CAD build for the part. Positions are in the model's coordinates, mm. A direction names the side the tool comes from. Round coordinates to 2 decimals unless told otherwise and drop trailing zeros. Loops run counter-clockwise (first coordinate to the right, second up) from the corner with the lowest first, then second, coordinate; pieces in that order, holes last.
```python
from build123d import *

# Parameters (mm, degrees)
SKETCH_1_W          = 40
SKETCH_1_H          = 2.5
EXTRUDE_1_DEPTH     = 18.5
SKETCH_2_R          = 1.5
CUT_EXTRUDE_1_DEPTH = 33.958808433
SKETCH_3_R          = 1.5
CUT_EXTRUDE_2_DEPTH = 40
SKETCH_4_W          = 40
SKETCH_4_H          = 5.719865779
CUT_EXTRUDE_3_DEPTH = 40
SKETCH_5_W          = 40
SKETCH_5_H          = 12.780134221
EXTRUDE_2_DEPTH     = 1
SKETCH_6_R          = 1.5
CUT_EXTRUDE_4_DEPTH = 31.221927206
SKETCH_8_W          = 40
SKETCH_8_H          = 3.5
EXTRUDE_3_DEPTH     = 5
SKETCH_9_R          = 3.8
CUT_EXTRUDE_5_DEPTH = 1
SKETCH_10_W         = 12
SKETCH_10_H         = 17.780134221
CUT_EXTRUDE_6_DEPTH = 1.5
CHAMFER_3_SIZE      = 0.7
CUT_EXTRUDE_7_DEPTH = 31.221927206
SKETCH_12_W         = 40
SKETCH_12_H         = 1.953894505
EXTRUDE_5_DEPTH     = 2
SKETCH_13_W         = 40
SKETCH_13_H         = 3.5
EXTRUDE_6_DEPTH     = 5
SKETCH_14_W         = 12
SKETCH_14_H         = 4.371099825
EXTRUDE_7_DEPTH     = 2
SKETCH_15_W         = 12
SKETCH_15_H         = 1.544999831
EXTRUDE_8_DEPTH     = 2


with BuildPart() as part:
    # Эскиз1 → Бобышка-Вытянуть1 (new body)
    with BuildSketch(Plane(origin=(0, 0, 0), x_dir=(1, 0, 0), z_dir=(0, 1, 0))):
        with Locations((7.162162162, 1.25)):
            Rectangle(SKETCH_1_W, SKETCH_1_H)
    extrude(amount=EXTRUDE_1_DEPTH)

    # Эскиз2 → Вырез-Вытянуть1 (cut, through all)
    with BuildSketch(Plane.XY):
        with Locations((-6.837837838, 3)):
            Circle(SKETCH_2_R)
        with Locations((21.162162162, 3)):
            Circle(SKETCH_2_R)
    extrude(amount=-CUT_EXTRUDE_1_DEPTH, mode=Mode.SUBTRACT)

    # Эскиз3 → Вырез-Вытянуть2 (cut)
    with BuildSketch(Plane.XY):
        with Locations((-2.337837838, 9.3)):
            Circle(SKETCH_3_R)
        with Locations((17.662162162, 9.3)):
            Circle(SKETCH_3_R)
    extrude(amount=-CUT_EXTRUDE_2_DEPTH, mode=Mode.SUBTRACT)

    # Эскиз4 → Вырез-Вытянуть3 (cut)
    with BuildSketch(Plane.XY):
        with Locations((7.162162162, 15.640067111)):
            Rectangle(SKETCH_4_W, SKETCH_4_H)
    extrude(amount=-CUT_EXTRUDE_3_DEPTH, mode=Mode.SUBTRACT)

    # Эскиз5 → Бобышка-Вытянуть2 (add)
    with BuildSketch(Plane.XY):
        with Locations((7.162162162, 6.390067111)):
            Rectangle(SKETCH_5_W, SKETCH_5_H)
    extrude(amount=EXTRUDE_2_DEPTH)

    # Эскиз6 → Вырез-Вытянуть4 (cut, through all)
    with BuildSketch(Plane(origin=(0, 0, -2.5), x_dir=(-1, 0, 0), z_dir=(0, 0, -1))):
        with Locations(Location((-17.662162162, 9.3, 0), (0, 0, 180))):
            Circle(SKETCH_6_R)
        with Locations(Location((2.337837838, 9.3, 0), (0, 0, 180))):
            Circle(SKETCH_6_R)
        with Locations(Location((6.837837838, 3, 0), (0, 0, 180))):
            Circle(SKETCH_6_R)
        with Locations(Location((-21.162162162, 3, 0), (0, 0, 180))):
            Circle(SKETCH_6_R)
    extrude(amount=-CUT_EXTRUDE_4_DEPTH, mode=Mode.SUBTRACT)

    # Эскиз8 → Бобышка-Вытянуть3 (add)
    with BuildSketch(Plane.XZ):
        with Locations((7.162162162, -0.75)):
            Rectangle(SKETCH_8_W, SKETCH_8_H)
    extrude(amount=EXTRUDE_3_DEPTH)

    # Эскиз9 → Вырез-Вытянуть5 (cut)
    with BuildSketch(Plane.XY.offset(1)):
        with Locations((-6.837837838, 3)):
            Circle(SKETCH_9_R)
        with Locations((21.162162162, 3)):
            Circle(SKETCH_9_R)
    extrude(amount=-CUT_EXTRUDE_5_DEPTH, mode=Mode.SUBTRACT)

    # Эскиз10 → Вырез-Вытянуть6 (cut)
    with BuildSketch(Plane(origin=(0, 0, -2.5), x_dir=(-1, 0, 0), z_dir=(0, 0, -1))):
        with Locations((-7.662162162, 3.890067111)):
            Rectangle(SKETCH_10_W, SKETCH_10_H)
    extrude(amount=-CUT_EXTRUDE_6_DEPTH, mode=Mode.SUBTRACT)

    # Фаска3
    chamfer_3_edges = [part.edges().sort_by_distance(p)[0] for p in [
        (-10.637837838, 3, 0),
        (17.362162162, 3, 0),
    ]]
    chamfer(chamfer_3_edges, length=CHAMFER_3_SIZE)

    # Эскиз11 → Вырез-Вытянуть7 (cut, through all)
    with BuildSketch(Plane.XY.offset(1)):
        Polygon((-12.837837838, 12.780134221), (-12.837837838, 7.280134221), (-7.337837838, 12.780134221), align=None)
        Polygon((27.162162162, 12.780134221), (21.662162162, 12.780134221), (27.162162162, 7.280134221), align=None)
    extrude(amount=-CUT_EXTRUDE_7_DEPTH, mode=Mode.SUBTRACT)

    # Эскиз12 → Бобышка-Вытянуть5 (add)
    with BuildSketch(Plane.XY.offset(1)):
        with Locations((7.162162162, 6.303186969)):
            Rectangle(SKETCH_12_W, SKETCH_12_H)
    extrude(amount=-EXTRUDE_5_DEPTH)

    # Эскиз13 → Бобышка-Вытянуть6 (add)
    with BuildSketch(Plane.XZ.offset(5)):
        with Locations((7.162162162, -0.75)):
            Rectangle(SKETCH_13_W, SKETCH_13_H)
    extrude(amount=EXTRUDE_6_DEPTH)

    # Эскиз14 → Бобышка-Вытянуть7 (add)
    with BuildSketch(Plane(origin=(0, 0, -2.5), x_dir=(-1, 0, 0), z_dir=(0, 0, -1))):
        with Locations((-7.662162162, -2.814450088)):
            Rectangle(SKETCH_14_W, SKETCH_14_H)
    extrude(amount=-EXTRUDE_7_DEPTH)

    # Эскиз15 → Бобышка-Вытянуть8 (add)
    with BuildSketch(Plane(origin=(0, 0, -2.5), x_dir=(-1, 0, 0), z_dir=(0, 0, -1))):
        with Locations((-7.662162162, 12.007634306)):
            Rectangle(SKETCH_15_W, SKETCH_15_H)
    extrude(amount=-EXTRUDE_8_DEPTH)


solid = part.part
```
Item 1: Cut at C-C, the plane z = -1.6. Give the cut face in (x, y), plus the area to 3 significant figures.
Answers follow:
outline: (-12.84, -10) - (27.16, -10) - (27.16, 7.28) - (21.66, 12.78) - (-7.34, 12.78) - (-12.84, 7.28) - close; hole circle Ø3 at (-6.84, 3); hole circle Ø3 at (-2.34, 9.3); hole (1.66, -0.63) - (13.66, -0.63) - (13.66, 11.24) - (1.66, 11.24) - close; hole circle Ø3 at (17.66, 9.3); hole circle Ø3 at (21.16, 3)
area: 710 mm2
Item 2: Cut at B-B, the plane x = 3. Give the cut face in (y, z), plus the area to 3 significant figures.
Answers follow:
outline: (-10, -2.5) - (-0.63, -2.5) - (-0.63, -1) - (11.24, -1) - (11.24, -2.5) - (12.78, -2.5) - (12.78, 1) - (-10, 1) - close
area: 61.9 mm2
Item 3: Cut at A-A, the plane y = 3. Give the cut face in (x, z), plus the area to 3 significant figures.
Answers follow:
outline: (-12.84, -2.5) - (-8.34, -2.5) - (-8.34, 0) - (-9.94, 0) - (-10.64, 0.7) - (-10.64, 1) - (-12.84, 1) - close; (-5.34, -2.5) - (1.66, -2.5) - (1.66, -1) - (13.66, -1) - (13.66, -2.5) - (19.66, -2.5) - (19.66, 0) - (18.06, 0) - (17.36, 0.7) - (17.36, 1) - (-3.04, 1) - (-3.04, 0.7) - (-3.74, 0) - (-5.34, 0) - close; (22.66, -2.5) - (27.16, -2.5) - (27.16, 1) - (24.96, 1) - (24.96, 0.7) - (24.26, 0) - (22.66, 0) - close
area: 92.8 mm2
Item 4: Flat gauge pin, fed straight in: P1, Ø9.5, axis at x = 7.5, y = 4.5, coming from the -Z side. Where does the tip first touch, or does it go through?
Answers follow:
P1: stops at z = -1
Item 5: Two-plate mould, pull along X, no slides. Class faces 4 (the flat face through (7, 12.78, -1)), 5 (the flat face through (8, 11.235, -2)), 6 (the flat face through (27.162, -1, -1)): released by +X, released by -X, zero draft, split by the parting line, or undercut.
Answers follow:
face 4: zero draft
face 5: undercut
face 6: released by +X
Item 6: 3-axis set-ups, long thin cutter, end or side, ignore diameter. For faces 1 (the flat face through (7, 2, 1)), 2 (the flat face through (8, -0.629, -2)), 3 (the flat face through (-7, 1, 0)): which of +Z, -Z, +X, -X, +Y, -Y reach the whole face in a straight line?
Answers follow:
face 1: +Z, +X, -X, +Y, -Y
face 2: -Z
face 3: +Z
Item 7: Cut at D-D, the plane y = 9.3. Give the cut face in (x, z).
Answers follow:
outline: (-10.82, -2.5) - (-3.84, -2.5) - (-3.84, 1) - (-10.82, 1) - close; (-0.84, -2.5) - (1.66, -2.5) - (1.66, -1) - (13.66, -1) - (13.66, -2.5) - (16.16, -2.5) - (16.16, 1) - (-0.84, 1) - close; (19.16, -2.5) - (25.14, -2.5) - (25.14, 1) - (19.16, 1) - close
Item 8: Probe line 1 (X direction, y = 3, z = 0.9); line 2 (X direction, y = 3, z = -1.05); line 3 (X direction, y = 3, z = -0.7). List the from-to ranges inside material, lowest first.
Answers follow:
line 1: x = -12.84 to -10.64, -3.04 to 17.36, 24.96 to 27.16
line 2: x = -12.84 to -8.34, -5.34 to 1.66, 13.66 to 19.66, 22.66 to 27.16
line 3: x = -12.84 to -8.34, -5.34 to 19.66, 22.66 to 27.16
